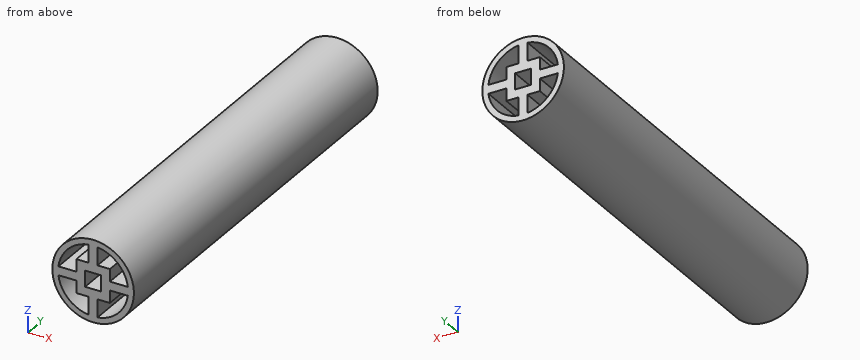
```python
from build123d import *

# Parameters (mm, degrees)
SKETCH1_R  = 14
SKETCH1_W  = 5.5
SKETCH1_H  = 5.5
BODY_DEPTH = 70


with BuildPart() as part:
    # Sketch1 → Body (new, symmetric)
    with BuildSketch(Plane(origin=(0, 0, 0), x_dir=(1, 0, 0), z_dir=(0, 1, 0))):
        with Locations(Location((0, 0, 0), (0, 0, 270))):
            Circle(SKETCH1_R)
        with BuildLine():
            Line((-5.75, 1.5), (-11.9058809, 1.5))
            ThreePointArc((-11.9058809, 1.5), (-8.485281374, 8.485281374), (-1.5, 11.9058809))
            Line((-1.5, 11.9058809), (-1.5, 5.75))
            Line((-1.5, 5.75), (-5.75, 5.75))
            Line((-5.75, 5.75), (-5.75, 1.5))
        make_face(mode=Mode.SUBTRACT)
        with BuildLine():
            Line((5.75, -5.75), (1.5, -5.75))
            Line((1.5, -5.75), (1.5, -11.9058809))
            ThreePointArc((1.5, -11.9058809), (8.485281374, -8.485281374), (11.9058809, -1.5))
            Line((11.9058809, -1.5), (5.75, -1.5))
            Line((5.75, -1.5), (5.75, -5.75))
        make_face(mode=Mode.SUBTRACT)
        with BuildLine():
            Line((5.75, 5.75), (1.5, 5.75))
            Line((1.5, 5.75), (1.5, 11.9058809))
            ThreePointArc((1.5, 11.9058809), (8.485281374, 8.485281374), (11.9058809, 1.5))
            Line((11.9058809, 1.5), (5.75, 1.5))
            Line((5.75, 1.5), (5.75, 5.75))
        make_face(mode=Mode.SUBTRACT)
        with BuildLine():
            Line((-5.75, -5.75), (-5.75, -1.5))
            Line((-5.75, -1.5), (-11.9058809, -1.5))
            ThreePointArc((-11.9058809, -1.5), (-8.485281374, -8.485281374), (-1.5, -11.9058809))
            Line((-1.5, -11.9058809), (-1.5, -5.75))
            Line((-1.5, -5.75), (-5.75, -5.75))
        make_face(mode=Mode.SUBTRACT)
        Rectangle(SKETCH1_W, SKETCH1_H, mode=Mode.SUBTRACT)
    extrude(amount=BODY_DEPTH, both=True)


solid = part.part
```
Build history of the part. All positions in model axes, mm. Round coordinates to 2 decimals unless told otherwise and drop trailing zeros. Loops run counter-clockwise (first coordinate to the right, second up) from the corner with the lowest first, then second, coordinate; pieces in that order, holes last.
Item 1: Pin check, flat tips, straight feed: P1, Ø7, axis at x = 7.5, y = -29.5, coming from the +Z side; P2, Ø4.5, axis at y = 30.5, z = 4.5, coming from the +X side; P3, Ø6, axis at x = -10.5, y = 33.5, coming from the +Z side; P4, Ø1.5, axis at x = -4, z = -7.5, coming from the +Y side. Stop position of each tip, or through.
Item 2: Drill centre lines: line 1 along Z through (x, y) = (-7, -37); line 2 along Z through (x, y) = (-6.5, 62); line 3 along X through (y, z) = (32, -2). Where is each one in solid material? Low to high.
Item 3: Saw through at A-A (z = 0). List the corners of the cut face in (x, y), then the cut area to 3 significant figures.
Item 4: Saw through at D-D (z = -10.5). List the corners of the cut face in (x, y), then the cut area to 3 significant figures.
Item 5: Saw through at C-C (y = -31). List the corners of the cut face in (x, z).
Item 6: Saw through at B-B (x = 0). List the corners of the cut face in (y, z).
Worked answers:
1. P1: stops at z = 13.42
1. P2: stops at x = 13.82
1. P3: stops at z = 11.82
1. P4: passes through
2. line 1: z = -12.12 to -9.75, -1.5 to 1.5, 9.75 to 12.12
2. line 2: z = -12.4 to -10.09, -1.5 to 1.5, 10.09 to 12.4
2. line 3: x = -13.86 to -11.83, -5.75 to -2.75, 2.75 to 5.75, 11.83 to 13.86
3. outline: (-14, -70) - (-2.75, -70) - (-2.75, 70) - (-14, 70) - close; (2.75, -70) - (14, -70) - (14, 70) - (2.75, 70) - close
3. area: 3,150 mm2
4. outline: (-9.26, -70) - (-5.81, -70) - (-5.81, 70) - (-9.26, 70) - close; (-1.5, -70) - (1.5, -70) - (1.5, 70) - (-1.5, 70) - close; (5.81, -70) - (9.26, -70) - (9.26, 70) - (5.81, 70) - close
4. area: 1,390 mm2
5. outline: circle Ø28 at (0, 0); hole (-11.91, -1.5) arc R12 ccw to (-1.5, -11.91) - (-1.5, -5.75) - (-5.75, -5.75) - (-5.75, -1.5) - close; hole (-11.91, 1.5) - (-5.75, 1.5) - (-5.75, 5.75) - (-1.5, 5.75) - (-1.5, 11.91) arc R12 ccw to start; hole (-2.75, -2.75) - (2.75, -2.75) - (2.75, 2.75) - (-2.75, 2.75) - close; hole (1.5, -11.91) arc R12 ccw to (11.91, -1.5) - (5.75, -1.5) - (5.75, -5.75) - (1.5, -5.75) - close; hole (1.5, 5.75) - (5.75, 5.75) - (5.75, 1.5) - (11.91, 1.5) arc R12 ccw to (1.5, 11.91) - close
6. outline: (-70, -14) - (70, -14) - (70, -2.75) - (-70, -2.75) - close; (-70, 2.75) - (70, 2.75) - (70, 14) - (-70, 14) - close
